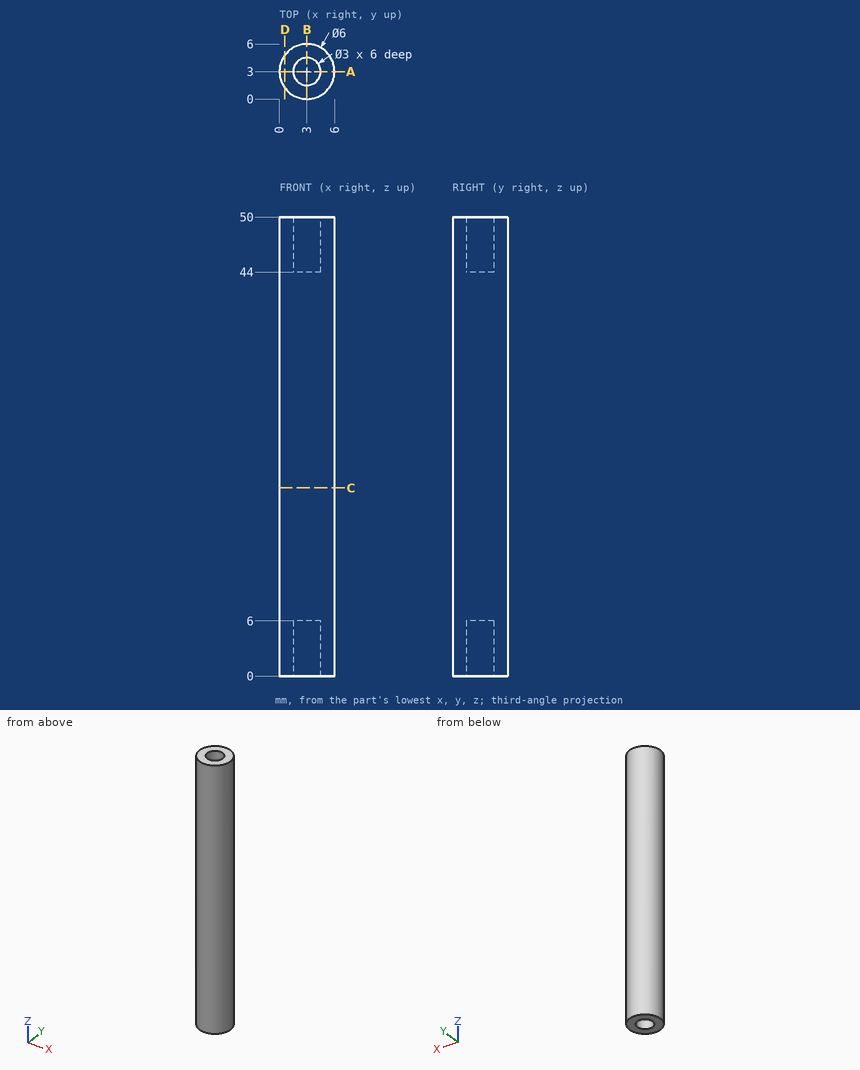
For this review, use the dimensioned drawing (mm, ordinates from the lowest corner) and the shaded views. Round coordinates to 2 decimals unless told otherwise and drop trailing zeros. Write each loop counter-clockwise with the first axis right and the second up, starting at its lowest first coordinate (ties: lowest second). Pieces come first, ordered by that corner, then holes. Notation, with made-up numbers: (72.5, -32) - (105.5, -32) arc R11 cw to (105.5, -27) - close; hole circle Ø9 at (86, 89.5). An arc over 180 degrees is marked (long way). Use a Markdown table: item, result.
Q1. Clearance check with flat-ended pins moving along their axes: pin 1 (1.8 mm diameter, centred on x = 3, y = 3, fed in from +Z); pin 2 (1.5 mm diameter, centred on x = 3, y = 3.5, fed in from -Z); pin 3 (3 mm diameter, centred on x = 5.5, z = 41, fed in from +Y). State where each tip first meets the part, or that it passes through.
Derived:
| item | result |
|---|---|
| pin 1 | stops at z = 44 |
| pin 2 | stops at z = 6 |
| pin 3 | stops at y = 5.83 |
Q2. Wall thickness on line 1 along Y through (x, z) = (3, 2.1); line 2 along Z through (x, y) = (3.3, 3); line 3 along X through (y, z) = (3.1, 21): over which ranges is each line inside the solid? List them lowest first.
Derived:
| item | result |
|---|---|
| line 1 | y = 0 to 1.5, 4.5 to 6 |
| line 2 | z = 6 to 44 |
| line 3 | x = 0 to 6 |
Q3. We need section D-D (x = 0.6). Give the boundary of the cut face in (y, z), plus the area to 3 significant figures.
Derived:
| item | result |
|---|---|
| outline | (1.2, 0) - (4.8, 0) - (4.8, 50) - (1.2, 50) - close |
| area | 180 mm2 |
Q4. We need section A-A (y = 3). Give the boundary of the cut face in (x, z).
Derived:
| item | result |
|---|---|
| outline | (0, 0) - (1.5, 0) - (1.5, 6) - (4.5, 6) - (4.5, 0) - (6, 0) - (6, 50) - (4.5, 50) - (4.5, 44) - (1.5, 44) - (1.5, 50) - (0, 50) - close |
Q5. We need section C-C (z = 20.5). Give the boundary of the cut face in (x, y), plus the area to 3 significant figures.
Derived:
| item | result |
|---|---|
| outline | circle Ø6 at (3, 3) |
| area | 28.3 mm2 |
